For this review, take the finished solid that the model builds, in its own axes (mm). A direction names the side the tool comes from. Give positions to 0.01 mm unless a question says otherwise; leave off trailing zeros. Write each loop counter-clockwise with the first axis right and the second up, starting at its lowest first coordinate (ties: lowest second). Pieces come first, ordered by that corner, then holes.
1) Draft analysis for pull direction X (two halves, no side actions). For faces 4 (the face through (-3.65, -9.24, -66.62)), 5 (the face through (-16.55, -41, -69)), 6 (the face through (6, -55, -58)), state which applies: pulls with the +X half, pulls with the -X half, needs draft (parallel to the pull), parting line crosses it, or undercut.
2) We need section D-D on z = -62.25. Give the boundary of the cut face in (x, y), and give its area (3 significant figures).
3) Machinability: for faces 1 (the face through (-17, -37, -65)), 2 (the face through (0, -37, -75)), 3 (the face through (15, -24, -65)), which of the approach directions +Z, -Z, +X, -X, +Y, -Y give a long, thin tool a straight path to every point of the face, cutting with its end or side? Answer none if there is none.
4) We need section C-C on y = -57.5. Give the boundary of the cut face in (x, z), and give its area (3 significant figures).
5) We need section A-A on x = 0. Give the boundary of the cut face in (y, z).
6) For P1, Ø1.4, axis at x = -17.5, y = -37.5, coming from the +Z side; P2, Ø2, axis at y = -35, z = -67, coming from the +X side; P3, Ø1, axis at x = -4.5, z = -68.5, coming from the +Y side, all flat-tipped, find the tip position at first contact; note any pin that passes through.
7) Wall thickness on line 1 along Y through (x, z) = (0, -60.5); line 2 along Z through (x, y) = (7.5, -57); line 3 along X through (y, z) = (-34.5, -61): over which ranges is each line inside the solid? List them lowest first.
8) We need section B-B on y = -37. Give the boundary of the cut face in (x, z).
from build123d import *

# Parameters (mm, degrees)
SKETCH025_W  = 34
SKETCH025_H  = 50
PAD023_DEPTH = 7.5
SKETCH017_R  = 18.25
PAD015_DEPTH = 7
SKETCH016_R  = 28
PAD014_DEPTH = 17


with BuildPart() as body026:
    # Sketch025 → Pad023 (new body)
    with BuildSketch(Plane.XY):
        with Locations((0.449597, -4.527582)):
            Rectangle(SKETCH025_W, SKETCH025_H)
    extrude(amount=PAD023_DEPTH)


with BuildPart() as body026_1:
    # Body026 placement: moved
    add(body026.part.moved(Location((0, -42, -72.5))))


with BuildPart() as body016:
    # Sketch017 → Pad015 (new body)
    with BuildSketch(Plane.XY.offset(2)):
        with Locations((0, -34)):
            Circle(SKETCH017_R)
    extrude(amount=PAD015_DEPTH)


with BuildPart() as body016_1:
    # Body016 placement: moved
    add(body016.part.moved(Location((0, -3, -67))))


with BuildPart() as bottom:
    # Sketch016 → Pad014 (new body)
    with BuildSketch(Plane.XY):
        with Locations((0, -34)):
            Circle(SKETCH016_R)
    extrude(amount=PAD014_DEPTH)


with BuildPart() as bottom_1:
    # Body015 placement: moved
    add(bottom.part.moved(Location((0, -3, -75))))

    # Cut034: cut Body016
    add(body016_1.part, mode=Mode.SUBTRACT)

    # Cut035: cut Body026
    add(body026_1.part, mode=Mode.SUBTRACT)


solid = bottom_1.part
Results list:
1. face 4: parting line crosses it
1. face 5: undercut
1. face 6: needs draft
2. outline: circle Ø56 at (0, -37); hole circle Ø36.5 at (0, -37)
2. area: 1,420 mm2
3. face 1: +Z
3. face 2: -Z, +X, -X, +Y, -Y
3. face 3: -Y
4. outline: (-19.07, -75) - (19.07, -75) - (19.07, -58) - (-19.07, -58) - close; hole (-16.55, -72.5) - (17.45, -72.5) - (17.45, -65) - (-16.55, -65) - close
4. area: 393 mm2
5. outline: (-65, -75) - (-9, -75) - (-9, -58) - (-18.75, -58) - (-18.75, -65) - (-21.53, -65) - (-21.53, -72.5) - (-65, -72.5) - close; (-65, -65) - (-55.25, -65) - (-55.25, -58) - (-65, -58) - close
6. P1: stops at z = -65
6. P2: stops at x = 27.98
6. P3: stops at y = -9.29
7. line 1: y = -65 to -55.25, -18.75 to -9
7. line 2: z = -75 to -72.5, -65 to -58
7. line 3: x = -27.89 to -18.08, 18.08 to 27.89
8. outline: (-28, -75) - (28, -75) - (28, -58) - (18.25, -58) - (18.25, -65) - (17.45, -65) - (17.45, -72.5) - (-16.55, -72.5) - (-16.55, -65) - (-18.25, -65) - (-18.25, -58) - (-28, -58) - close
